Can you work these out from the drawing? Everything is in mm from the part's minimum corner. A direction names the side the tool comes from. Give positions to 0.01 mm unless a question says otherwise; leave off trailing zeros. Write each loop counter-clockwise with the first axis right and the second up, starting at its lowest first coordinate (ties: lowest second). Pieces come first, ordered by that corner, then holes. Notation, with made-up numbers: (35.5, -18) - (67.5, -18) arc R20 ccw to (67.5, 6) - close; hole circle Ø11 at (-31, 46.25). An arc over 180 degrees is marked (long way). Answer in a Markdown table with one row per item.
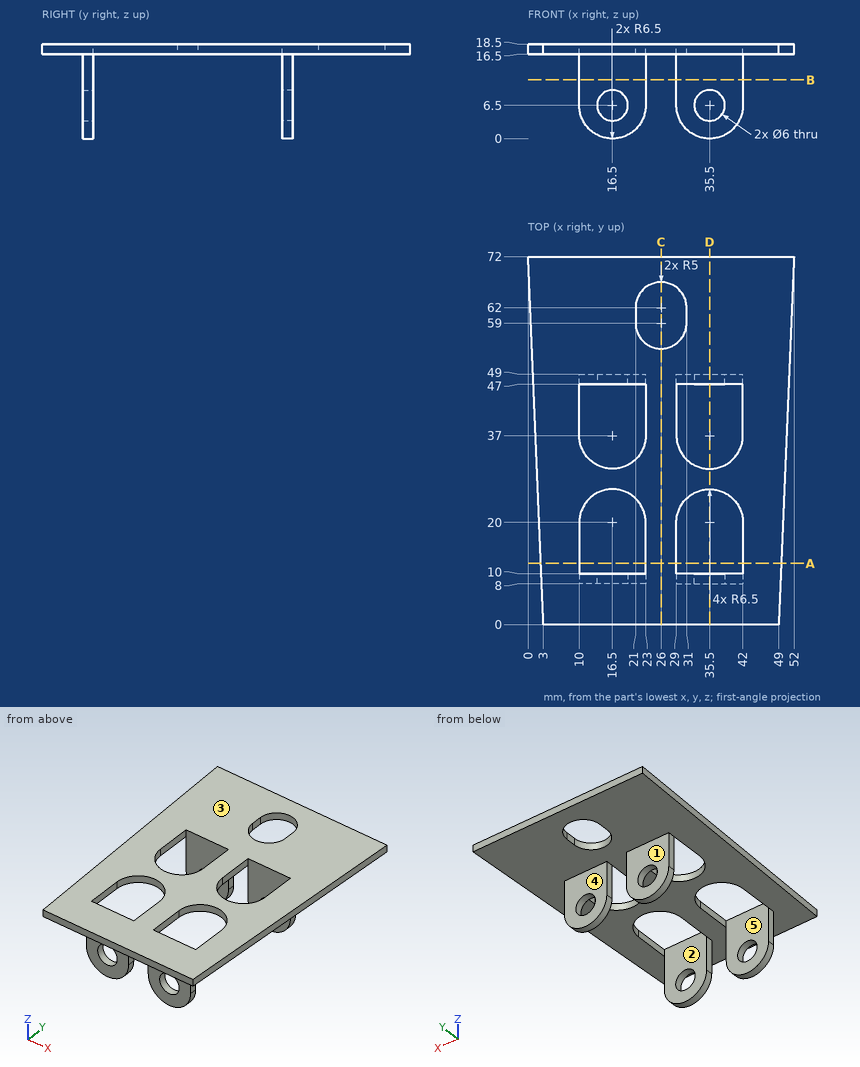
1) If I drill on line 1 (Y direction, x = 13, z = 1.5); line 2 (Z direction, x = 35.5, y = 48.55); line 3 (Z direction, x = 46, y = 35), over which ranges is the centre line in solid material (lowest first)?
Check values:
| item | result |
|---|---|
| line 1 | y = 8 to 10, 47 to 49 |
| line 2 | z = 0 to 3.5, 9.5 to 18.5 |
| line 3 | z = 16.5 to 18.5 |
2) Will these pins go through, and if not, where does the flat tip stop? P1, Ø2, axis at y = 41, z = 17.5, coming from the +X side; P2, Ø1.6, axis at y = 42.5, z = 18, coming from the +X side; P3, Ø0.6, axis at y = 40, z = 17.5, coming from the -X side.
Check values:
| item | result |
|---|---|
| P1 | stops at x = 50.75 |
| P2 | stops at x = 50.8 |
| P3 | stops at x = 1.32 |
3) Imagine slicing it at C-C (x = 26). List the corners of the cut face in (y, z) for me, then the cut area to 3 significant figures.
Check values:
| item | result |
|---|---|
| outline | (0, 16.5) - (54, 16.5) - (54, 18.5) - (0, 18.5) - close; (67, 16.5) - (72, 16.5) - (72, 18.5) - (67, 18.5) - close |
| area | 118 mm2 |
4) On a 3-axis mill with a long thin cutter (end or side, diameter ignored), from which of +Z, -Z, +X, -X, +Y, -Y can I reach the whole of each face in a straight line? I mean the marked faces 4 and 5. Say none if no direction works.
Check values:
| item | result |
|---|---|
| face 4 | -Z, +X, -X, +Y |
| face 5 | +Z, -Z |
5) We'd pull the mould along Y, two halves only. Please class the marked faces 1, 2 and 3: +Y half, -Y half, draft (parallel to the pull), parting line (faces both ways), or undercut.
Check values:
| item | result |
|---|---|
| face 1 | +Y half |
| face 2 | undercut |
| face 3 | draft |
6) Imagine slicing it at D-D (x = 35.5). List the corners of the cut face in (y, z) for me, then the cut area to 3 significant figures.
Check values:
| item | result |
|---|---|
| outline | (0, 16.5) - (8, 16.5) - (8, 9.5) - (10, 9.5) - (10, 18.5) - (0, 18.5) - close; (8, 0) - (10, 0) - (10, 3.5) - (8, 3.5) - close; (26.5, 16.5) - (30.5, 16.5) - (30.5, 18.5) - (26.5, 18.5) - close; (47, 0) - (49, 0) - (49, 3.5) - (47, 3.5) - close; (47, 9.5) - (49, 9.5) - (49, 16.5) - (72, 16.5) - (72, 18.5) - (47, 18.5) - close |
| area | 120 mm2 |
7) Imagine slicing it at A-A (y = 12). List the corners of the cut face in (x, z) for me.
Check values:
| item | result |
|---|---|
| outline | (2.5, 16.5) - (10, 16.5) - (10, 18.5) - (2.5, 18.5) - close; (23, 16.5) - (29, 16.5) - (29, 18.5) - (23, 18.5) - close; (42, 16.5) - (49.5, 16.5) - (49.5, 18.5) - (42, 18.5) - close |
8) Imagine slicing it at B-B (z = 11.5). List the corners of the cut face in (x, y) for me, then the cut area to 3 significant figures.
Check values:
| item | result |
|---|---|
| outline | (10, 8) - (23, 8) - (23, 10) - (10, 10) - close; (10, 47) - (23, 47) - (23, 49) - (10, 49) - close; (29, 8) - (42, 8) - (42, 10) - (29, 10) - close; (29, 47) - (42, 47) - (42, 49) - (29, 49) - close |
| area | 104 mm2 |
